The listing builds one solid part. Answer for the finished solid, in the listing's coordinates (mm). A direction names the side the tool comes from. Round coordinates to 2 decimals unless told otherwise and drop trailing zeros. Order: outer loops, then holes, each group sorted by start corner. A loop starts at its lowest first (then second) coordinate and runs counter-clockwise, first axis right, second up. Notation, with made-up numbers: (84.5, -18) - (93.5, -18) arc R7 ccw to (93.5, -14) - close; hole circle Ø3 at (38, -37.75). An arc over 180 degrees is marked (long way). Use CSV: the item, a comma, the result in double quotes. Start each with the question number.
Item 1: Find section A-A, the plane z = 14. Give the vertices of the cut face in (x, y), plus the area to 3 significant figures.
Item 2: Straight lines are drawn through the part: line 1 along Y through (x, z) = (0, 8); line 2 along Y through (x, z) = (0, 19); line 3 along X through (y, z) = (-4.5, 20.5). For each, find the intervals that lie inside material, in ascending order. Write a range as [from, to].
Item 3: Find section B-B, the plane y = -3. Give the vertices of the cut face in (x, z), plus the area to 3 significant figures.
Item 4: Determine the mould class of faces 4 (the flat face through (2, -1, 0)), 5 (the cylindrical face through (-3, -3.4, 14.8)), 6 (the flat face through (7.34, -4.02, 14.79)) for opening direction Y: +Y half, -Y half, draft (parallel to the pull), parting line (faces both ways), or undercut.
Item 5: For faces 1 (the flat face through (0, 3, 21)), 2 (the cylindrical face through (4.59, -7.36, 14.79)), 3 (the flat face through (0, 3, 9)), determine the directions among +Z, -Z, +X, -X, +Y, -Y from which every point of the face is accessible in a straight line to the end or side of a thin tool.
Item 6: Find section C-C, the plane x = 0. Give the vertices of the cut face in (y, z), plus the area to 3 significant figures.
Item 7: Find section D-D, the plane z = 4.5. Give the vertices of the cut face in (x, y), plus the area to 3 significant figures.
Item 8: Flat-ended cylindrical pins translate along their axes: P1, Ø5, axis at x = -6, y = 4, coming from the -Z side; P2, Ø1, axis at x = -6.5, z = 18, coming from the +Y side; P3, Ø1.8, axis at x = -1.5, y = 2, coming from the +Z side; P4, Ø5.5, axis at x = 0, y = -3.5, coming from the -Z side. Find the tip coordinate at first contact, or state that the pin passes through.
```python
from build123d import *

# Parameters (mm, degrees)
STOCK_AUGET_1_OUTLINE_R = 3
STOCK_AUGET_1_DEPTH     = 30
ESQUISSE1_W             = 7
ESQUISSE1_H             = 12
BOSS_EXTRU_1_DEPTH      = 6


# Read off the part's stored shape, not the designer's step: Stock-auget-1
with BuildPart() as part:
    # Stock-auget-1 outline → Stock-auget-1 (new body)
    with BuildSketch(Plane.XY):
        with BuildLine():
            ThreePointArc((8.256781031, -2.464537089), (9.916165038, -0.760058008), (12.17539903, -0.015298993))
            Line((12.17539903, -0.015298993), (-12.563147232, -9.56e-07))
            ThreePointArc((-12.563147232, -9.56e-07), (-10.082691958, -0.660415437), (-8.256781031, -2.464537089))
            Line((-8.256781031, -2.464537089), (-6.450006579, -5.535462911))
            ThreePointArc((-6.450006579, -5.535462911), (-4.622753843, -7.340352207), (-2.140548629, -8))
            Line((-2.140548629, -8), (2.140548629, -8))
            ThreePointArc((2.140548629, -8), (4.622753843, -7.340352207), (6.450006579, -5.535462911))
            Line((6.450006579, -5.535462911), (8.256781031, -2.464537089))
        make_face()
        with Locations((0, -3.5)):
            Circle(STOCK_AUGET_1_OUTLINE_R, mode=Mode.SUBTRACT)
    extrude(amount=STOCK_AUGET_1_DEPTH)

    # Esquisse1 → Boss.-Extru.1 (add)
    with BuildSketch(Plane(origin=(-4.805e-06, -0.007770331, 0), x_dir=(0.9999998088216733, -0.0006183499145584942, 0), z_dir=(0.0006183499145584943, 0.9999998088216734, 0))):
        with Locations((-0.193144829, -15)):
            Rectangle(ESQUISSE1_W, ESQUISSE1_H)
    extrude(amount=BOSS_EXTRU_1_DEPTH)


solid = part.part
```
Worked out:
1,outline,"(-12.56, 0) arc R5 cw to (-8.26, -2.46) - (-6.45, -5.54) arc R5 ccw to (-2.14, -8) - (2.14, -8) arc R5 ccw to (6.45, -5.54) - (8.26, -2.46) arc R5 cw to (12.18, -0.02) - (3.31, -0.01) - (3.31, 5.99) - (-3.69, 5.99) - (-3.69, -0.01) - close; hole circle Ø6 at (0, -3.5)"
1,area,"131 mm²"
2,line 1,"y = [-8, -6.5], [-0.5, -0.01]"
2,line 2,"y = [-8, -6.5], [-0.5, 5.99]"
2,line 3,"x = [-7.06, -2.83], [2.83, 7.06]"
3,outline,"(-7.94, 0) - (-2.96, 0) - (-2.96, 30) - (-7.94, 30) - close; (2.96, 0) - (7.94, 0) - (7.94, 30) - (2.96, 30) - close"
3,area,"299 mm²"
4,face 4,"draft"
4,face 5,"undercut"
4,face 6,"-Y half"
5,face 1,"+Z, +X, -X, +Y"
5,face 2,"+Z, -Z, +X, -Y"
5,face 3,"-Z, +X, -X, +Y"
6,outline,"(-8, 0) - (-6.5, 0) - (-6.5, 30) - (-8, 30) - close; (-0.5, 0) - (-0.01, 0) - (-0.01, 9) - (5.99, 9) - (5.99, 21) - (-0.01, 21) - (-0.01, 30) - (-0.5, 30) - close"
6,area,"132 mm²"
7,outline,"(-12.56, 0) arc R5 cw to (-8.26, -2.46) - (-6.45, -5.54) arc R5 ccw to (-2.14, -8) - (2.14, -8) arc R5 ccw to (6.45, -5.54) - (8.26, -2.46) arc R5 cw to (12.18, -0.02) - close; hole circle Ø6 at (0, -3.5)"
7,area,"89.2 mm²"
8,P1,"stops at z = 9"
8,P2,"stops at y = 0"
8,P3,"stops at z = 21"
8,P4,"passes through"
